from build123d import *

# Parameters (mm, degrees)
F0_R     = 11.1125
F1_DEPTH = 457.2
F2_W     = 165.1
F2_H     = 11.1125
F2_W_2   = 19.05
F2_H_2   = 6.35
F3_DEPTH = 12.7


with BuildPart() as f1:
    # F0 (on Front) → F1 (new body)
    with BuildSketch(Plane.XZ):
        Circle(F0_R)
    extrude(amount=F1_DEPTH)

    # F2 (on Right) → F3 (cut, symmetric)
    with BuildSketch(Plane.YZ):
        with Locations((-374.65, -5.55625)):
            Rectangle(F2_W, F2_H)
        Polygon((-457.2, 11.1125), (-457.2, 0), (-431.8, 11.1125), align=None)
        Rectangle(F2_W_2, F2_H_2)
    extrude(amount=F3_DEPTH, both=True, mode=Mode.SUBTRACT)


solid = f1.part
Geometry check sheet. Reference: the model listing, model coordinates, mm. A direction names the side the tool comes from. Coordinates: 2 decimals unless noted, no trailing zeros. Order: outer loops, then holes, each group sorted by start corner. A loop starts at its lowest first (then second) coordinate and runs counter-clockwise, first axis right, second up. Notation, with made-up numbers: (-29.5, 0.25) - (-15.5, 0.25) arc R12 ccw to (-15.5, 12.25) - close; hole circle Ø9 at (-36.5, 75). An arc over 180 degrees is marked (long way). Answer in a Markdown table with one row per item. Add a question column.
1) Set-up check for faces 5 (the flat face through (0, 0, -6)), 6 (the flat face through (0, -376, 0)): record each of +Z, -Z, +X, -X, +Y, -Y from which the full face is reachable in a straight line by a thin tool's end or side.
2) Release check for a two-part mould opening along Z. For faces 1 (the flat face through (0, -5, 3.175)), 2 (the flat face through (-0.156, -447.5, 4.244)), 3 (the flat face through (0, -5, -3.175)), 4 (the flat face through (0, 0, 6)) record: +Z half, -Z half, draft (parallel to the pull), parting line (faces both ways), or undercut.
3) Gauge pin test, flat ends, axial feed: P1, Ø6.5, axis at x = 2, y = -381, coming from the -Z side; P2, Ø5, axis at x = -3, y = -215.5, coming from the -Z side; P3, Ø1.9, axis at x = 4.5, z = -1, coming from the +Y side (3 decimals). Record the tip position at first contact, or that the pin passes through.
4) Cross-section at C-C, the plane y = -426.5. Record the cut outline in (x, z) (1 decimal), then the cut area to 3 significant figures.
5) Cross-section at A-A, the plane x = 0. Record the cut outline in (y, z) (1 decimal), then the cut area to 4 significant figures.
6) Material ranges on line 1 along Y through (x, z) = (-9, -0.25) (3 decimals); line 2 along Y through (x, z) = (4, -9.5); line 3 along X through (y, z) = (-223, 1), recorded low to high. Write a range as [from, to].
7) Cross-section at B-B, the plane y = -54.5. Record the cut outline in (x, z) (1 decimal), then the cut area to 3 significant figures.
Check result:
| question | item | result |
|---|---|---|
| 1 | face 5 | +Z, -Z, +X, -X, +Y |
| 1 | face 6 | -Z, +X, -X, -Y |
| 2 | face 1 | undercut |
| 2 | face 2 | +Z half |
| 2 | face 3 | undercut |
| 2 | face 4 | draft |
| 3 | P1 | stops at z = 0 |
| 3 | P2 | stops at z = -11.1 |
| 3 | P3 | stops at y = -9.525 |
| 4 | outline | (-11.1, 0) - (11.1, 0) arc R11.1 ccw to start |
| 4 | area | 194 mm² |
| 5 | outline | (-457.2, 0) - (-292.1, 0) - (-292.1, -11.1) - (0, -11.1) - (0, -3.2) - (-9.5, -3.2) - (-9.5, 3.2) - (0, 3.2) - (0, 11.1) - (-431.8, 11.1) - close |
| 5 | area | 8,125 mm² |
| 6 | line 1 | y = [-292.1, -9.525] |
| 6 | line 2 | y = [-292.1, 0] |
| 6 | line 3 | x = [-11.07, 11.07] |
| 7 | outline | circle Ø22.2 at (0, 0) |
| 7 | area | 388 mm² |
